from build123d import *

# Parameters (mm, degrees)
F3_DEPTH       = 26
F3_DEPTH_BACK  = 0.2
F5_D           = 6
F9_D           = 3.3
F9_DEPTH       = 15
F9_CSINK_D     = 4.5
F9_CSINK_ANGLE = 90
F9_TIP         = 0.9914200214


with BuildPart() as f1:
    # F0 (on Front) → F1 (revolve)
    with BuildSketch(Plane.XZ):
        Polygon((77.5, 21), (77.5, 18), (82.5, 18), (82.5, 0), (92.5, 0), (92.5, 79), (82.5, 79), (82.5, 56), (77.5, 56), (77.5, 53), (68.5, 53), (68.5, 21), align=None)
    revolve(axis=Axis((0, 0, 27.8796814382), (0, 0, -1)))

    # F2 (on face) → F3 (cut, two sides)
    with BuildSketch(Plane.XY.offset(53)) as f3_sk:
        with BuildLine():
            Line((50, -10), (75, -10))
            ThreePointArc((75, -10), (85, 0), (75, 10))
            Line((75, 10), (50, 10))
            Line((50, 10), (50, -10))
        make_face()
        with BuildLine():
            Line((-16.3397459622, 48.3012701892), (-28.8397459622, 69.9519052838))
            ThreePointArc((-28.8397459622, 69.9519052838), (-42.5, 73.6121593217), (-46.1602540378, 59.9519052838))
            Line((-46.1602540378, 59.9519052838), (-33.6602540378, 38.3012701892))
            Line((-33.6602540378, 38.3012701892), (-16.3397459622, 48.3012701892))
        make_face()
        with BuildLine():
            Line((-33.6602540378, -38.3012701892), (-46.1602540378, -59.9519052838))
            ThreePointArc((-46.1602540378, -59.9519052838), (-42.5, -73.6121593217), (-28.8397459622, -69.9519052838))
            Line((-28.8397459622, -69.9519052838), (-16.3397459622, -48.3012701892))
            Line((-16.3397459622, -48.3012701892), (-33.6602540378, -38.3012701892))
        make_face()
    extrude(amount=F3_DEPTH, mode=Mode.SUBTRACT)
    extrude(f3_sk.sketch, amount=-F3_DEPTH_BACK, mode=Mode.SUBTRACT)

    # F5 (through all)
    with Locations(Plane.XY.offset(52.8)):
        with Locations((75, 0), (-37.5, 64.9519052838), (-37.5, -64.9519052838)):
            Hole(F5_D / 2)

    # F6 (on Front) → F7 (revolve, cut)
    with BuildSketch(Plane.XZ):
        Polygon((-95, 52), (-95, 37), (-65, 37), (-65, 44.5), (-90, 44.5), (-90, 52), align=None)
    revolve(axis=Axis((-80, 0, 37), (1, 0, 0)), mode=Mode.SUBTRACT)

    # F9
    with Locations(Plane.XY.offset(79)):
        with Locations((-87.5, 0), (-54.5553576626, 68.410254716), (19.4705817212, 85.3061923159), (78.8347759415, 37.9648271728), (78.8347759415, -37.9648271728), (19.4705817212, -85.3061923159), (-54.5553576626, -68.410254716)):
            CounterSinkHole(F9_D / 2, F9_CSINK_D / 2, depth=F9_DEPTH, counter_sink_angle=F9_CSINK_ANGLE)
            with Locations((0, 0, -(F9_DEPTH + F9_TIP / 2))):  # 118° drill point
                Cone(0, F9_D / 2, F9_TIP, mode=Mode.SUBTRACT)


solid = f1.part
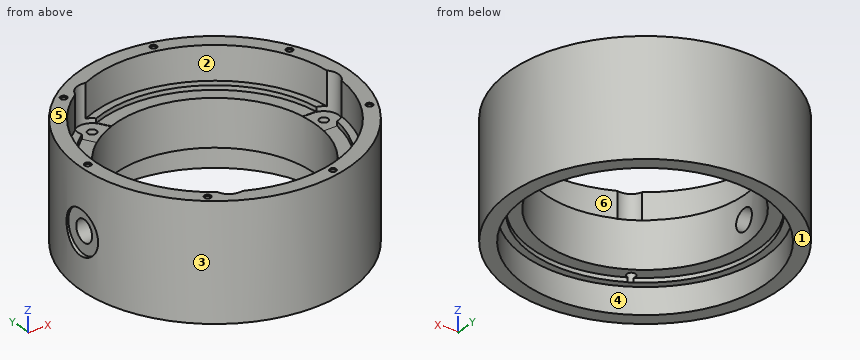
Design review of the part built by this model. Coordinates are the model's own, in mm. Face numbers are marked on the shaded views. A direction names the side the tool comes from. Round coordinates to 2 decimals unless told otherwise and drop trailing zeros. Write each loop counter-clockwise with the first axis right and the second up, starting at its lowest first coordinate (ties: lowest second). Pieces come first, ordered by that corner, then holes. Notation, with made-up numbers: (44, -8.75) -> (54, -8.75) arc R17 ccw to (54, 11.25) -> close; hole circle Ø11 at (8, 48.25). An arc over 180 degrees is marked (long way). One line per question, with ' | ' between items.
(1) Take a section at A-A, the plane x = 0. State the section outline as (y, z) points.
Result sheet:
outline: (-92.5, 0) -> (-82.5, 0) -> (-82.5, 18) -> (-77.5, 18) -> (-77.5, 21) -> (-68.5, 21) -> (-68.5, 53) -> (-77.5, 53) -> (-77.5, 56) -> (-82.5, 56) -> (-82.5, 79) -> (-92.5, 79) -> close; (68.5, 21) -> (77.5, 21) -> (77.5, 18) -> (82.5, 18) -> (82.5, 0) -> (92.5, 0) -> (92.5, 79) -> (82.5, 79) -> (82.5, 56) -> (77.5, 56) -> (77.5, 53) -> (68.5, 53) -> close
(2) Take a section at B-B, the plane z = 37. State the section outline as (x, y) points.
Result sheet:
outline: (-91.28, -15) arc R92.5 ccw (long way) to (-91.28, 15) -> (-90, 15) -> (-90, 7.5) -> (-68.09, 7.5) arc R68.5 cw (long way) to (-68.09, -7.5) -> (-90, -7.5) -> (-90, -15) -> close; hole circle Ø6 at (-37.5, -64.95); hole circle Ø6 at (-37.5, 64.95); hole circle Ø6 at (75, 0)
(3) Take a section at D-D, the plane y = 80. State the section outline as (x, z) points, and give its area (3 significant figures).
Result sheet:
outline: (-46.44, 0) -> (-20.16, 0) -> (-20.16, 18) -> (20.16, 18) -> (20.16, 0) -> (46.44, 0) -> (46.44, 79) -> (20.16, 79) -> (20.16, 56) -> (-20.16, 56) -> (-20.16, 79) -> (-46.44, 79) -> close | area: 5,680 mm2
(4) Take a section at C-C, the plane z = 11. State the section outline as (x, y) points, and give its area (3 significant figures).
Result sheet:
outline: circle Ø185 at (0, 0); hole circle Ø165 at (0, 0) | area: 5,500 mm2
(5) Wall thickness on line 1 (X direction, y = 0, z = 75.75); line 2 (X direction, y = 0, z = 7); line 3 (Z direction, x = 73.5, y = -4.5): over which ranges is each line inside the solid? List them lowest first. Write a range as [from, to].
Result sheet:
line 1: [-92.5, -89.15], [-85.85, -82.5], [85, 92.5] | line 2: [-92.5, -82.5], [82.5, 92.5] | line 3: [21, 52.8]
(6) Insertion check: P1, Ø10, axis at x = -28, z = 50.5, coming from the +Y side; P2, Ø1, axis at y = 5.5, z = 61.5, coming from the -X side; P3, Ø8, axis at x = 54.5, y = 48.5, coming from the +Z side; P4, Ø5.5, axis at x = -37.5, y = -64.95, coming from the -Z side. Each pin has a flat end and moves straight along its axis. Give the tip position at first contact, or say it passes through.
Result sheet:
P1: y = 89.59 | P2: x = -92.36 | P3: z = 53 | P4: through
(7) Draft analysis for pull direction X (two halves, no side actions). For the marked faces 1, 2 and 3, state which applies: released by +X, released by -X, zero draft, split by the parting line, or undercut.
Result sheet:
face 1: zero draft | face 2: undercut | face 3: split by the parting line
(8) Machinability: for the marked faces 4, 5 and 6, which of the approach directions +Z, -Z, +X, -X, +Y, -Y give a long, thin tool a straight path to every point of the face, cutting with its end or side? Answer none if there is none.
Result sheet:
face 4: -Z | face 5: +Z, +X, -X, +Y, -Y | face 6: +Z
